The model under review builds one solid part; all positions refer to its coordinate system, in mm. A direction names the side the tool comes from. Round coordinates to 2 decimals unless told otherwise and drop trailing zeros. Order: outer loops, then holes, each group sorted by start corner. A loop starts at its lowest first (then second) coordinate and runs counter-clockwise, first axis right, second up.
1) Consider section C-C (z = 53.5). Give the boundary of the cut face in (x, y), then the cut area to 3 significant figures.
2) To check wall thickness, follow L1, parallel to X at y = -9.05, z = 0; L2, parallel to X at y = 0.7, z = 0; L3, parallel to Y at x = -6, z = -37.5. State the ranges of each line that lie inside material, in increasing order.
3) Consider section D-D (x = 14.5). Give the boundary of the cut face in (y, z), then the cut area to 3 significant figures.
4) Consider section B-B (x = -28). Give the boundary of the cut face in (y, z).
5) Mouldability with a two-part tool opening along Z and no side actions: class faces 1 (the face through (0, -10, 15)), 2 (the face through (3.755, -8.986, 11.923)), 3 (the face through (-33.71, -4.93, -4.43)), 4 (the face through (-14, -8, 0)) as pulls with the +Z half, pulls with the -Z half, needs draft (parallel to the pull), parting line crosses it, or undercut.
6) Clearance check with flat-ended pins moving along their axes: P1, Ø10, axis at x = 48.5, z = 17, coming from the -Y side; P2, Ø2.5, axis at x = -75, z = 0, coming from the +Y side; P3, Ø1.5, axis at x = -46.5, y = -0.5, coming from the +Z side; P4, Ø5, axis at x = -8.5, y = 0.5, coming from the -Z side. State where each tip first meets the part, or that it passes through.
7) Consider section A-A (y = -5). Give the boundary of the cut face in (x, z).
8) Machinability: for faces 5 (the face through (-31.24, -2.42, -6.94)), 6 (the face through (-34, 3, -1)), 7 (the face through (-34.2, 0, -1.1)), which of the approach directions +Z, -Z, +X, -X, +Y, -Y give a long, thin tool a straight path to every point of the face, cutting with its end or side? Answer none if there is none.
from build123d import *

# Parameters (mm, degrees)
SKETCH_1_R          = 79.5
SKETCH_1_R_2        = 1.6
EXTRUDE_1_DEPTH     = 3
SKETCH_5_R          = 34
EXTRUDE_2_DEPTH     = 10
CUT_EXTRUDE_START   = -22
SKETCH_7_R          = 1.6
CUT_EXTRUDE_1_DEPTH = 22
SKETCH_8_R          = 32
CUT_EXTRUDE_2_DEPTH = 11
SKETCH_10_R         = 12.5
CUT_EXTRUDE_3_DEPTH = 12


with BuildPart() as part:
    # 草图1 → 凸台-拉伸1 (new body)
    with BuildSketch(Plane(origin=(0, 0, 0), x_dir=(1, 0, 0), z_dir=(0, 1, 0))):
        with Locations(Location((0, 0, 0), (0, 0, 270))):
            Circle(SKETCH_1_R)
        with Locations(Location((0, 75, 0), (0, 0, 270))):
            Circle(SKETCH_1_R_2, mode=Mode.SUBTRACT)
        with Locations(Location((75, 0, 0), (0, 0, 270))):
            Circle(SKETCH_1_R_2, mode=Mode.SUBTRACT)
        with Locations(Location((0, -75, 0), (0, 0, 270))):
            Circle(SKETCH_1_R_2, mode=Mode.SUBTRACT)
        with Locations(Location((-75, 0, 0), (0, 0, 270))):
            Circle(SKETCH_1_R_2, mode=Mode.SUBTRACT)
        with Locations(Location((0, 21.92, 0), (0, 0, 270))):
            Circle(SKETCH_1_R_2, mode=Mode.SUBTRACT)
        with Locations(Location((21.92, 0, 0), (0, 0, 270))):
            Circle(SKETCH_1_R_2, mode=Mode.SUBTRACT)
        with Locations(Location((0, -21.92, 0), (0, 0, 270))):
            Circle(SKETCH_1_R_2, mode=Mode.SUBTRACT)
        with Locations(Location((-21.92, 0, 0), (0, 0, 270))):
            Circle(SKETCH_1_R_2, mode=Mode.SUBTRACT)
    extrude(amount=EXTRUDE_1_DEPTH)

    # 草图5 → 凸台-拉伸2 (add)
    with BuildSketch(Plane.XZ):
        with Locations(Location((0, 0, 0), (0, 0, 90))):
            Circle(SKETCH_5_R)
    extrude(amount=EXTRUDE_2_DEPTH)

    # 草图7 → 切除-拉伸1 (cut)
    with BuildSketch(Plane(origin=(0, 3, 0), x_dir=(1, 0, 0), z_dir=(0, 1, 0)).offset(CUT_EXTRUDE_START)):
        with Locations(Location((0, 21.92, 0), (0, 0, 90))):
            Circle(SKETCH_7_R)
        with Locations(Location((21.92, 0, 0), (0, 0, 90))):
            Circle(SKETCH_7_R)
        with Locations(Location((0, -21.92, 0), (0, 0, 90))):
            Circle(SKETCH_7_R)
        with Locations(Location((-21.92, 0, 0), (0, 0, 90))):
            Circle(SKETCH_7_R)
    extrude(amount=CUT_EXTRUDE_1_DEPTH, mode=Mode.SUBTRACT)

    # 草图8 → 切除-拉伸2 (cut)
    with BuildSketch(Plane(origin=(0, 3, 0), x_dir=(1, 0, 0), z_dir=(0, 1, 0))):
        with Locations(Location((0, 0, 0), (0, 0, 270))):
            Circle(SKETCH_8_R)
    extrude(amount=-CUT_EXTRUDE_2_DEPTH, mode=Mode.SUBTRACT)

    # 草图10 → 切除-拉伸3 (cut)
    with BuildSketch(Plane(origin=(0, -8, 0), x_dir=(1, 0, 0), z_dir=(0, 1, 0))):
        with Locations(Location((0, 0, 0), (0, 0, 270))):
            Circle(SKETCH_10_R)
    extrude(amount=-CUT_EXTRUDE_3_DEPTH, mode=Mode.SUBTRACT)


solid = part.part
Answer below:
1. outline: (-58.8, 0) - (58.8, 0) - (58.8, 3) - (-58.8, 3) - close
1. area: 353 mm2
2. L1: x = -34 to -23.52, -20.32 to -12.5, 12.5 to 20.32, 23.52 to 34
2. L2: x = -79.5 to -76.6, -73.4 to -32, 32 to 73.4, 76.6 to 79.5
2. L3: y = 0 to 3
3. outline: (-10, -30.75) - (0, -30.75) - (0, -78.17) - (3, -78.17) - (3, -28.53) - (-8, -28.53) - (-8, 28.53) - (3, 28.53) - (3, 78.17) - (0, 78.17) - (0, 30.75) - (-10, 30.75) - close
3. area: 456 mm2
4. outline: (-10, -19.29) - (0, -19.29) - (0, -74.41) - (3, -74.41) - (3, -15.49) - (-8, -15.49) - (-8, 15.49) - (3, 15.49) - (3, 74.41) - (0, 74.41) - (0, 19.29) - (-10, 19.29) - close
5. face 1: needs draft
5. face 2: undercut
5. face 3: parting line crosses it
5. face 4: undercut
6. P1: stops at y = 0
6. P2: passes through
6. P3: stops at z = 64.88
6. P4: stops at z = -79.27
7. outline: circle Ø68 at (0, 0); hole circle Ø64 at (0, 0)
8. face 5: +Y
8. face 6: +Z, -Z, +X, -X, +Y
8. face 7: -Y
